Can you work these out from the drawing? Everything is in mm from the part's minimum corner. A direction names the side the tool comes from. Coordinates: 2 decimals unless noted, no trailing zeros. Order: outer loops, then holes, each group sorted by start corner. A loop starts at its lowest first (then second) coordinate and runs counter-clockwise, first axis right, second up. Notation, with made-up numbers: (27.25, 89.25) - (39.25, 89.25) arc R22 cw to (39.25, 112.25) - close; hole circle Ø7 at (84, 65.5). An arc over 180 degrees is marked (long way). Use CSV: the item, a comma, the result in double quotes. Start each with the question number.
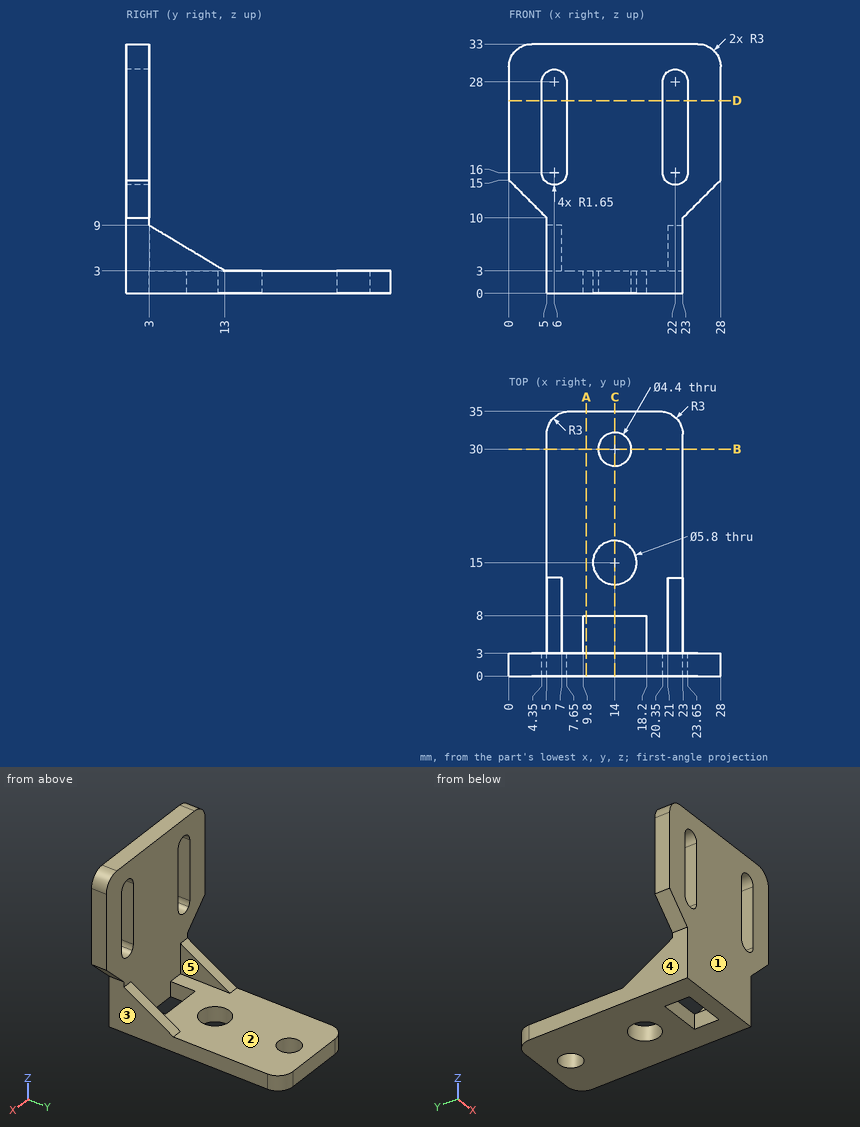
Item 1: Suppose I cut it at B-B on y = 30. Write out the boundary of the cut face in (x, z).
Item 2: For the marked faces 1 and 2, which set-ups out of +Z, -Z, +X, -X, +Y, -Y let a thin tool reach every point of the face, with its end or its side?
Item 3: Suppose I cut it at D-D on z = 25.5. Write out the boundary of the cut face in (x, y).
Item 4: Suppose I cut it at A-A on x = 10.25. Write out the boundary of the cut face in (y, z), then the cut area to 3 significant figures.
Item 5: We'd pull the mould along X, two halves only. Please class the marked faces 3, 4 and 5: released by +X, released by -X, zero draft, split by the parting line, or undercut.
Item 6: Suppose I cut it at C-C on x = 14. Write out the boundary of the cut face in (y, z).
Item 7: For pin 1 Ø0.9 at (y, z) = (5.5, 1) entering from +X; pin 2 Ø2.5 at (y, z) = (5, 2) entering from -X; pin 3 Ø10 at (x, z) = (11, 29.5) entering from +Y; pin 4 Ø4 at (x, y) = (14, 30) entering from +Z, each with a flat end and sliding along its axis, tell me the tip position at first contact or that it passes through.
Item 8: Please list where these lines run through material, in increasing order: line 1 along Y through (x, z) = (14, 1.75); line 2 along Y through (x, z) = (17.75, 31). Write a range as from..to.
Here are the results:
1,outline,"(5, 0) - (11.8, 0) - (11.8, 3) - (5, 3) - close; (16.2, 0) - (23, 0) - (23, 3) - (16.2, 3) - close"
2,face 1,"+Z, -Z, +X, -X, -Y"
2,face 2,"+Z, +Y"
3,outline,"(0, 0) - (4.35, 0) - (4.35, 3) - (0, 3) - close; (7.65, 0) - (20.35, 0) - (20.35, 3) - (7.65, 3) - close; (23.65, 0) - (28, 0) - (28, 3) - (23.65, 3) - close"
4,outline,"(0, 0) - (3, 0) - (3, 33) - (0, 33) - close; (8, 0) - (35, 0) - (35, 3) - (8, 3) - close"
4,area,"180 mm^2"
5,face 3,"released by +X"
5,face 4,"released by -X"
5,face 5,"undercut"
6,outline,"(0, 0) - (3, 0) - (3, 33) - (0, 33) - close; (8, 0) - (12.1, 0) - (12.1, 3) - (8, 3) - close; (17.9, 0) - (27.8, 0) - (27.8, 3) - (17.9, 3) - close; (32.2, 0) - (35, 0) - (35, 3) - (32.2, 3) - close"
7,pin 1,"x = 23"
7,pin 2,"x = 5"
7,pin 3,"y = 3"
7,pin 4,"through"
8,line 1,"0..3, 8..12.1, 17.9..27.8, 32.2..35"
8,line 2,"0..3"
